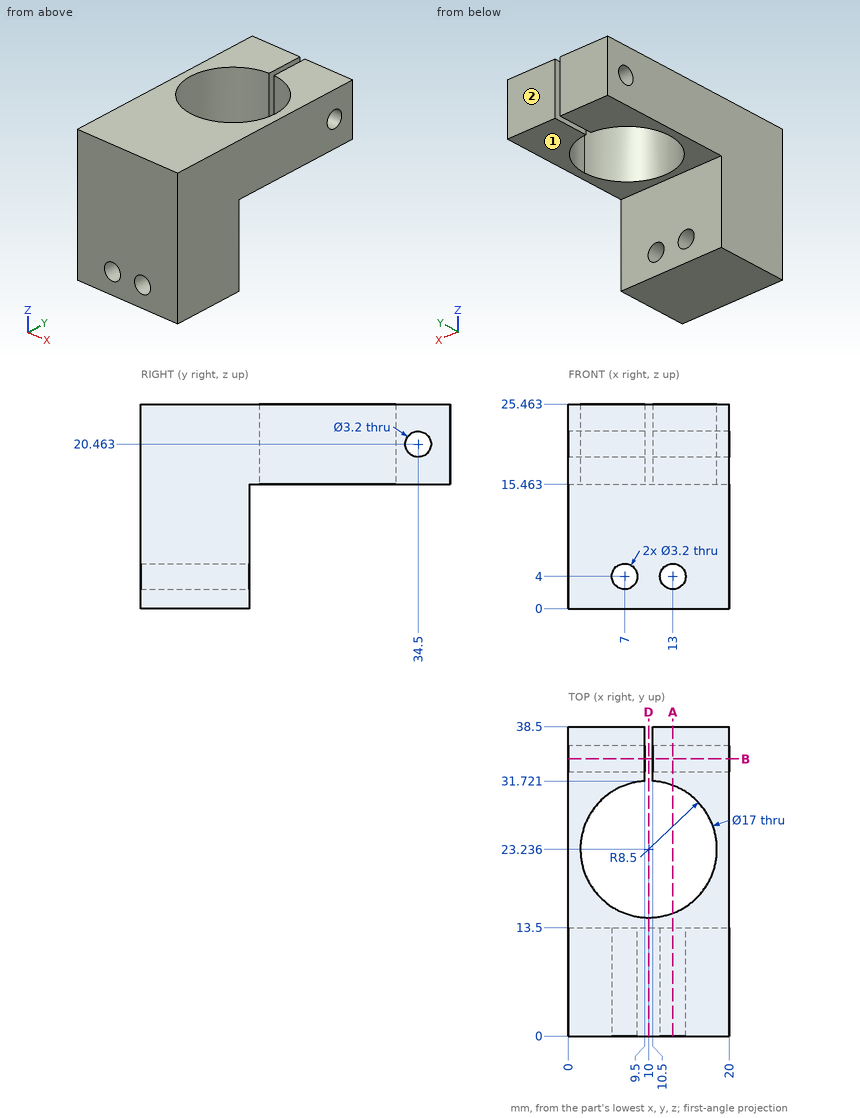
Answer from the drawing. Dimensions are ordinates in mm from the lowest x, y and z of the part. A direction names the side the tool comes from. Give positions to 0.01 mm unless a question says otherwise; leave off trailing zeros. Write each loop counter-clockwise with the first axis right and the second up, starting at its lowest first coordinate (ties: lowest second). Pieces come first, ordered by that corner, then holes.
1) Section D-D (x = 10) is taken. Write down the section's boundary in (y, z) (1 decimal), and give its area (3 significant figures).
2) Section B-B (y = 34.5) is taken. Write down the section's boundary in (x, z).
3) Find the intervals of material crossed by L1, parallel to Z at x = 7, y = 9; L2, parallel to Z at x = 13.25, y = 34.5; L3, parallel to X at y = 33, z = 16, in increasing order.
4) Section A-A (x = 13) is taken. Write down the section's boundary in (y, z).
5) A tool of negligible diameter and unlimited length cuts with its end or side. For the marked faces 1 and 2, from which of +Z, -Z, +X, -X, +Y, -Y can it reach the whole face along a straight path? Write none if from no direction.
Response:
1. outline: (0, 0) - (13.5, 0) - (13.5, 15.5) - (14.7, 15.5) - (14.7, 25.5) - (0, 25.5) - close
1. area: 356 mm2
2. outline: (0, 15.46) - (9.5, 15.46) - (9.5, 18.86) - (0, 18.86) - close; (0, 22.06) - (9.5, 22.06) - (9.5, 25.46) - (0, 25.46) - close; (10.5, 15.46) - (20, 15.46) - (20, 18.86) - (10.5, 18.86) - close; (10.5, 22.06) - (20, 22.06) - (20, 25.46) - (10.5, 25.46) - close
3. L1: z = 0 to 2.4, 5.6 to 25.46
3. L2: z = 15.46 to 18.86, 22.06 to 25.46
3. L3: x = 0 to 9.5, 10.5 to 20
4. outline: (0, 0) - (13.5, 0) - (13.5, 2.4) - (0, 2.4) - close; (0, 5.6) - (13.5, 5.6) - (13.5, 15.46) - (15.28, 15.46) - (15.28, 25.46) - (0, 25.46) - close; (31.19, 15.46) - (38.5, 15.46) - (38.5, 25.46) - (31.19, 25.46) - close; hole circle Ø3.2 at (34.5, 20.46)
5. face 1: -Z, +X, -X, +Y
5. face 2: +Z, -Z, +X, -X, +Y
